Geometry check sheet. Reference: drawing and pictorial views, mm from the part's lowest x, y, z. A direction names the side the tool comes from. Round coordinates to 2 decimals unless told otherwise and drop trailing zeros. Loops run counter-clockwise (first coordinate to the right, second up) from the corner with the lowest first, then second, coordinate; pieces in that order, holes last. Notation, with made-up numbers: (2, 44) -> (23, 44) arc R13 cw to (23, 52) -> close; hole circle Ø6 at (69.5, 60). An arc over 180 degrees is marked (long way). Use one line per item in the form item = value.
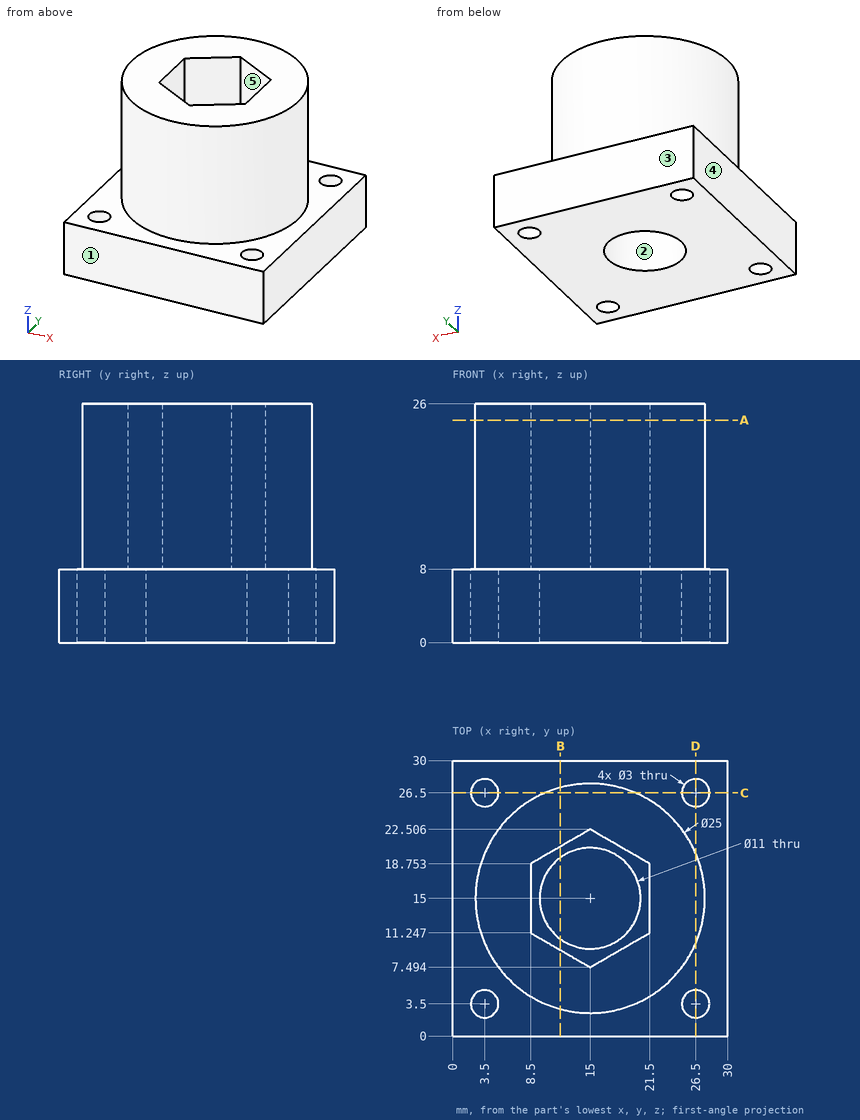
1. Tool access check on the marked faces 4 and 5. Record the directions out of +Z, -Z, +X, -X, +Y, -Y that give a thin tool (end or side, any length) a straight path to the whole face; none if there is none.
Return value:
face_4 = +Z, -Z, -X, +Y, -Y
face_5 = +Z
2. Section check C-C (y = 26.5). Record the boundary of the cut face in (x, z).
Return value:
outline = (0, 0) -> (2, 0) -> (2, 8) -> (0, 8) -> close; (5, 0) -> (25, 0) -> (25, 8) -> (19.9, 8) -> (19.9, 26) -> (10.1, 26) -> (10.1, 8) -> (5, 8) -> close; (28, 0) -> (30, 0) -> (30, 8) -> (28, 8) -> close
3. Material ranges on line 1 along Y through (x, z) = (26.5, 3.25); line 2 along Y through (x, z) = (15, 17) (1 decimal); line 3 along Z through (x, y) = (24.75, 25.5), recorded low to high.
Return value:
line_1 = 0 to 2, 5 to 25, 28 to 30
line_2 = 2.5 to 7.5, 22.5 to 27.5
line_3 = 0 to 8
4. Section check B-B (x = 11.75). Record the boundary of the cut face in (y, z), then the cut area to 3 significant figures.
Return value:
outline = (0, 0) -> (10.56, 0) -> (10.56, 8) -> (9.37, 8) -> (9.37, 26) -> (2.93, 26) -> (2.93, 8) -> (0, 8) -> close; (19.44, 0) -> (30, 0) -> (30, 8) -> (27.07, 8) -> (27.07, 26) -> (20.63, 26) -> (20.63, 8) -> (19.44, 8) -> close
area = 401 mm2
5. Gauge pin test, flat ends, axial feed: pin 1 (2.5 mm diameter, centred on y = 14.5, z = 14, fed in from +X); pin 2 (2 mm diameter, centred on x = 8.5, z = 22.5, fed in from -Y) (1 decimal); pin 3 (4 mm diameter, centred on y = 10.5, z = 14.5, fed in from -X). Record the tip position at first contact, or that the pin passes through.
Return value:
pin_1 = 27.5
pin_2 = 3.8
pin_3 = 2.75
6. Section check A-A (z = 24.25). Record the boundary of the cut face in (x, y) (1 decimal).
Return value:
outline = circle Ø25 at (15, 15); hole (8.5, 11.2) -> (15, 7.5) -> (21.5, 11.2) -> (21.5, 18.8) -> (15, 22.5) -> (8.5, 18.8) -> close
7. Mould release check, pull along Y, two halves, no side actions. Record for the marked faces 1, 2 and 3: released by +Y, released by -Y, zero draft, split by the parting line, or undercut.
Return value:
face_1 = released by -Y
face_2 = undercut
face_3 = released by +Y
